Read the model definition and answer for the solid it produces. Units are mm, in the model's axes. A direction names the side the tool comes from. Round coordinates to 2 decimals unless told otherwise and drop trailing zeros. Write each loop counter-clockwise with the first axis right and the second up, starting at its lowest first coordinate (ties: lowest second). Pieces come first, ordered by that corner, then holes. Notation, with made-up numbers: (-7, -22.75) -> (36, -22.75) arc R32 ccw to (36, 7.25) -> close; hole circle Ø5 at (72, 10.25). An arc over 180 degrees is marked (long way). Return JSON: item names as keys, results as strings.
Autodesk Inventor part; units mm, degrees
ref_plane "YZ Plane" through (0, 0, 0) normal (1, 0, 0) x (0, 1, 0)
ref_plane "XZ Plane" through (0, 0, 0) normal (0, 1, 0) x (-1, 0, 0)
ref_plane "XY Plane" through (0, 0, 0) normal (0, 0, 1) x (1, 0, 0)
sketch "Sketch1" plane through (0, 0, 0) normal (0, 0, 1) x (1, 0, 0)
  arc A0 (12, -5) -> (-12, -5) centre (0, 0) ccw
  line L0 (0, 0) -> (0, -5)
  line L1 (-12, -5) -> (-17, -5)
  line L2 (-17, -5) -> (-17, 16)
  line L3 (0, -5) -> (17, -5)
  line L4 (17, -5) -> (17, 16)
  line L5 (17, 16) -> (-17, 16)
  dimension "d0" = 26
  dimension "d1" = 5
  dimension "d2" = 17
  dimension "d3" = 21
  dimension "d4" = 17
  dimension "d5" = 21
extrude "Extrusion1" add sketch "Sketch1" along normal blind 25
ref_plane "Work Plane1" through (0, 0, 0) normal (0, -1, 0) x (1, 0, 0)
sketch "Sketch2" plane through (0, 0, 0) normal (0, -1, 0) x (1, 0, 0)
  line L0 (0, 0) -> (0, 25)
  line L1 (-13, 25) -> (13, 25)
  line L2 (0, 12.5) -> (-13, 12.5)
  line L3 (-13, 12.5) -> (-15, 12.5)
  line L4 (-15, 12.5) -> (-15, 16.5)
  line L5 (-15, 16.5) -> (-13.5, 16.5)
  line L6 (-13.5, 16.5) -> (-13.5, 20.5)
  line L7 (-13.5, 20.5) -> (-16.5, 20.5)
  line L8 (-16.5, 20.5) -> (-16.5, 16.5)
  line L9 (-16.5, 16.5) -> (-15, 16.5)
  line L10 (-15, 12.5) -> (-15, 8.5)
  line L11 (-15, 8.5) -> (-13.5, 8.5)
  line L12 (-13.5, 8.5) -> (-13.5, 4.5)
  line L13 (-13.5, 4.5) -> (-16.5, 4.5)
  line L14 (-16.5, 4.5) -> (-16.5, 8.5)
  line L15 (-16.5, 8.5) -> (-15, 8.5)
  line L16 (13, 12.5) -> (15, 12.5)
  line L17 (15, 12.5) -> (15, 16.5)
  line L18 (15, 16.5) -> (13.5, 16.5)
  line L19 (13.5, 16.5) -> (13.5, 20.5)
  line L20 (13.5, 20.5) -> (16.5, 20.5)
  line L21 (16.5, 20.5) -> (16.5, 16.5)
  line L22 (16.5, 16.5) -> (15, 16.5)
  line L23 (15, 12.5) -> (15, 8.5)
  line L24 (15, 8.5) -> (13.5, 8.5)
  line L25 (13.5, 8.5) -> (13.5, 4.5)
  line L26 (13.5, 4.5) -> (16.5, 4.5)
  line L27 (16.5, 4.5) -> (16.5, 8.5)
  line L28 (16.5, 8.5) -> (15, 8.5)
  point P0 (-12, 25)
  point P1 (12, 25)
  dimension "d8" = 2
  dimension "d9" = 4
  dimension "d10" = 1.5
  dimension "d11" = 4
  dimension "d12" = 3
  dimension "d13" = 4
revolve "Revolution1" cut sketch "Sketch2" angle 180 about axis through (0, 0, 0) along (0, 0, -1)
equation "\"BendRadius\" = Thickness"
equation "\"BendReliefWidth\" = Thickness"
equation "\"BendReliefDepth\" = 0.5 * Thickness"
equation "\"CornerReliefSize\" = 4 * Thickness"
equation "\"MinimumRemnant\" = 2 * Thickness"
equation "\"TransitionRadius\" = BendRadius"
equation "\"JacobiRadiusSize\" = BendRadius"
equation "\"GapSize\" = Thickness"
properties part number "abrazadera_smps"
Item 1: Flat-ended cylindrical pins translate along their axes: pin 1 (5 mm diameter, centred on x = -6, z = 11, fed in from -Y); pin 2 (3 mm diameter, centred on x = 8, y = 10, fed in from +Z); pin 3 (8 mm diameter, centred on x = -7.5, z = 13.5, fed in from -Y). Find the tip coordinate at first contact, or state that the pin passes through.
Worked answers:
{"pin 1": "stops at y = 9.84", "pin 2": "stops at z = 25", "pin 3": "stops at y = 6.06"}
Item 2: Section C-C (x = 0) is taken. Give the vertices of the cut face in (y, z), then the cut area to 3 significant figures.
Worked answers:
{"outline": "(13, 0) -> (16, 0) -> (16, 4.5) -> (13.5, 4.5) -> (13.5, 8.5) -> (16, 8.5) -> (16, 16.5) -> (13.5, 16.5) -> (13.5, 20.5) -> (16, 20.5) -> (16, 25) -> (13, 25) -> close", "area": "55.0 mm2"}
Item 3: Section A-A (y = 0) is taken. Give the vertices of the cut face in (x, z), then the cut area to 3 significant figures.
Worked answers:
{"outline": "(-17, 0) -> (-13, 0) -> (-13, 25) -> (-17, 25) -> close; (13, 0) -> (17, 0) -> (17, 25) -> (13, 25) -> close; hole (-16.5, 4.5) -> (-13.5, 4.5) -> (-13.5, 8.5) -> (-16.5, 8.5) -> close; hole (-16.5, 16.5) -> (-13.5, 16.5) -> (-13.5, 20.5) -> (-16.5, 20.5) -> close; hole (13.5, 4.5) -> (16.5, 4.5) -> (16.5, 8.5) -> (13.5, 8.5) -> close; hole (13.5, 16.5) -> (16.5, 16.5) -> (16.5, 20.5) -> (13.5, 20.5) -> close", "area": "152 mm2"}
Item 4: For a pull along Y with two mould halves and no side action, classify faces 3 (the flat face through (0, 16, 12)), 4 (the cylindrical face through (-14.507, 7.862, 18.472)), 5 (the flat face through (14, -5, 12)) as released by +Y, released by -Y, zero draft, split by the parting line, or undercut.
Worked answers:
{"face 3": "released by +Y", "face 4": "undercut", "face 5": "released by -Y"}
Item 5: A tool of negligible diameter and unlimited length cuts with its end or side. For faces 1 (the flat face through (0, 14, 16.5)), 2 (the flat face through (-4, 13, 25)), from which of +Z, -Z, +X, -X, +Y, -Y can it reach the whole face along a straight path? Write none if from no direction.
Worked answers:
{"face 1": "none", "face 2": "+Z, +X, -X, +Y, -Y"}
Item 6: Straight lines are drawn through the part: L1, parallel to X at y = 0, z = 7.75; L2, parallel to Z at x = -9, y = 11; L3, parallel to X at y = 0, z = 14.5. For each, find the intervals that lie inside material, in ascending order. Write a range as [from, to].
Worked answers:
{"L1": "x = [-17, -16.5], [-13.5, -13], [13, 13.5], [16.5, 17]", "L2": "z = [0, 4.5], [8.5, 16.5], [20.5, 25]", "L3": "x = [-17, -13], [13, 17]"}
Item 7: Section D-D (x = 7.5) is taken. Give the vertices of the cut face in (y, z), then the cut area to 3 significant figures.
Worked answers:
{"outline": "(10.62, 0) -> (16, 0) -> (16, 25) -> (10.62, 25) -> close; hole (11.22, 4.5) -> (14.7, 4.5) -> (14.7, 8.5) -> (11.22, 8.5) -> close; hole (11.22, 16.5) -> (14.7, 16.5) -> (14.7, 20.5) -> (11.22, 20.5) -> close", "area": "107 mm2"}
Item 8: Section B-B (z = 7.75) is taken. Give the vertices of the cut face in (x, y).
Worked answers:
{"outline": "(-17, -5) -> (-15.72, -5) arc R16.5 cw to (-4.03, 16) -> (-17, 16) -> close; (-12.54, -5) -> (-12, -5) arc R13 cw (long way) to (12, -5) -> (12.54, -5) arc R13.5 ccw (long way) to start; (4.03, 16) arc R16.5 cw to (15.72, -5) -> (17, -5) -> (17, 16) -> close"}
